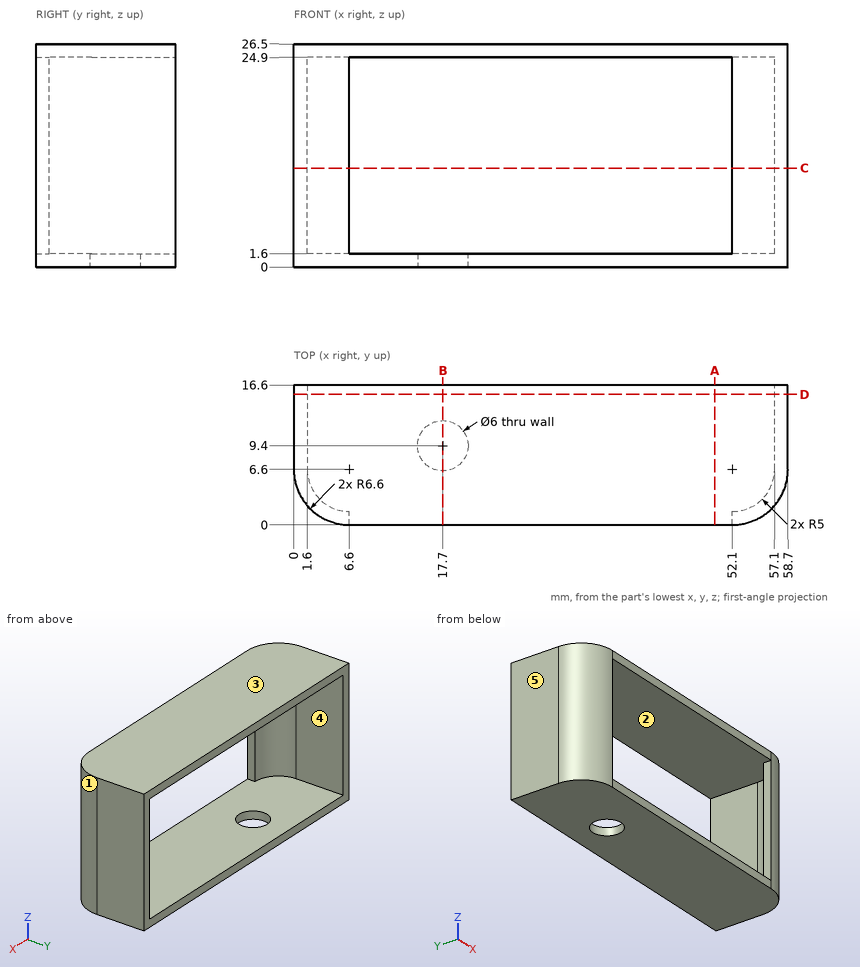
Source: three-view drawing plus pictorial views. Frame: mm from the lowest corner of the part. A direction names the side the tool comes from. Coordinates: 2 decimals unless noted, no trailing zeros. Order: outer loops, then holes, each group sorted by start corner. A loop starts at its lowest first (then second) coordinate and runs counter-clockwise, first axis right, second up. Notation, with made-up numbers: (38.5, 16.5) -> (57.5, 16.5) arc R13 ccw to (57.5, 32.5) -> close; hole circle Ø7 at (-16.75, 79). An arc over 180 degrees is marked (long way). Write item = value, one per line.
(1) Cut plane C-C on z = 11.75. Return loops of the section in (x, y), plus the area to 3 significant figures.
Solved:
outline = (0, 6.6) arc R6.6 ccw to (6.6, 0) -> (6.6, 1.6) arc R5 cw to (1.6, 6.6) -> (1.6, 16.6) -> (0, 16.6) -> close; (52.1, 0) arc R6.6 ccw to (58.7, 6.6) -> (58.7, 16.6) -> (57.1, 16.6) -> (57.1, 6.6) arc R5 cw to (52.1, 1.6) -> close
area = 61.2 mm²
(2) Pin query (flat end, axial travel): pin 1 Ø0.8 at (y, z) = (1, 15.5) entering from -X; pin 2 Ø0.8 at (y, z) = (1, 8) entering from +X; pin 3 Ø12 at (x, z) = (12.5, 15.5) entering from +Y. Return the tip coordinate at first contact, or that it passes through.
Solved:
pin_1 = 2.54
pin_2 = 56.16
pin_3 = 1.6
(3) Cut plane D-D on y = 15.5. Return loops of the section in (x, z).
Solved:
outline = (0, 0) -> (58.7, 0) -> (58.7, 26.5) -> (0, 26.5) -> close; hole (1.6, 1.6) -> (57.1, 1.6) -> (57.1, 24.9) -> (1.6, 24.9) -> close
(4) Pull-direction query (X, two-part tool) for the marked faces 3, 4 and 5; classes: pulls with the +X half, pulls with the -X half, needs draft (parallel to the pull), parting line crosses it, or undercut.
Solved:
face_3 = needs draft
face_4 = undercut
face_5 = pulls with the -X half
(5) Access query for the marked faces 1 and 2. Directions: +Z, -Z, +X, -X, +Y, -Y. A direction counts if a zero-diameter tool reaches every point of the face in a straight line with its end or side. Return the directions, or none.
Solved:
face_1 = +Z, -Z, +X, -Y
face_2 = +Y
(6) Cut plane A-A on x = 50. Return loops of the section in (y, z).
Solved:
outline = (0, 0) -> (16.6, 0) -> (16.6, 1.6) -> (0, 1.6) -> close; (0, 24.9) -> (16.6, 24.9) -> (16.6, 26.5) -> (0, 26.5) -> close
(7) Line query: line 1 (Z direction, x = 45, y = 6.25); line 2 (Y direction, x = 17.7, z = 0.75); line 3 (X direction, y = 11.5, z = 4). Output: solid intervals per line, ascending.
Solved:
line_1 = 0 to 1.6, 24.9 to 26.5
line_2 = 0 to 6.4, 12.4 to 16.6
line_3 = 0 to 1.6, 57.1 to 58.7
(8) Cut plane B-B on x = 17.7. Return loops of the section in (y, z).
Solved:
outline = (0, 0) -> (6.4, 0) -> (6.4, 1.6) -> (0, 1.6) -> close; (0, 24.9) -> (16.6, 24.9) -> (16.6, 26.5) -> (0, 26.5) -> close; (12.4, 0) -> (16.6, 0) -> (16.6, 1.6) -> (12.4, 1.6) -> close
